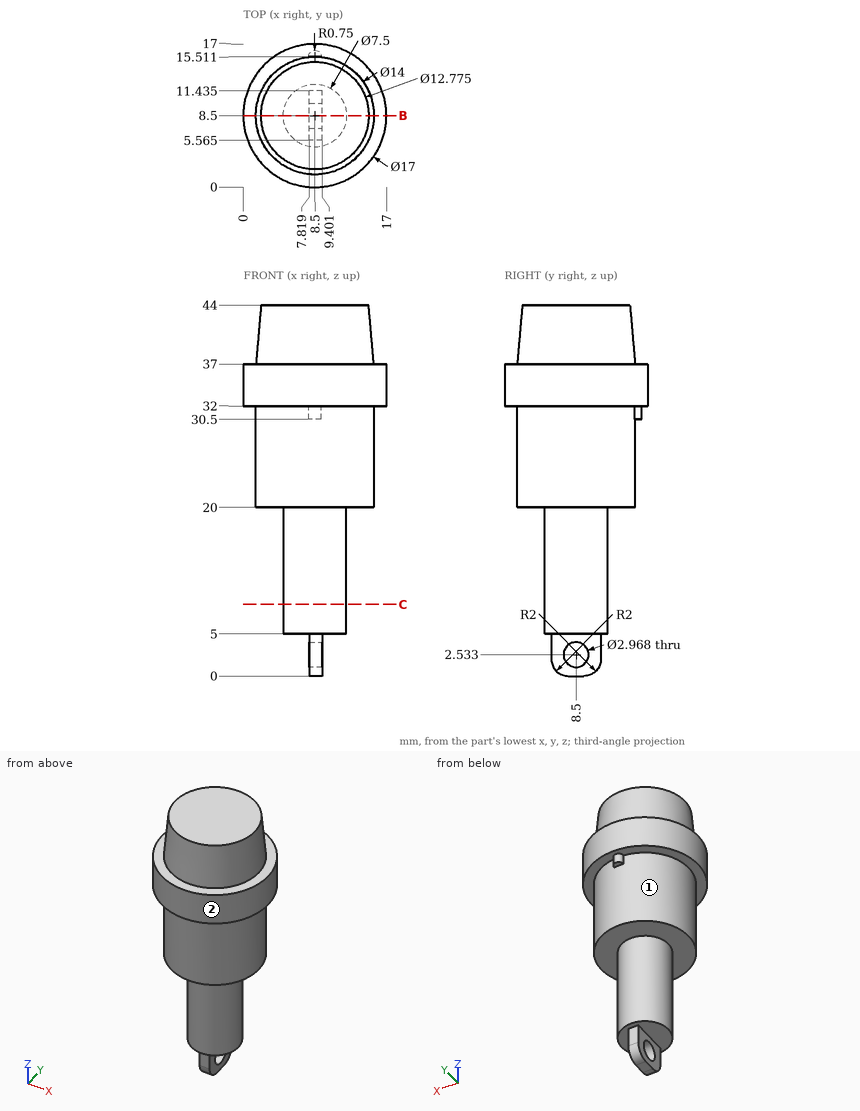
Print and shaded views of the part. All mm, measured from the part's lowest x, y and z. A direction names the side the tool comes from. Round coordinates to 2 decimals unless told otherwise and drop trailing zeros. Order: outer loops, then holes, each group sorted by start corner. A loop starts at its lowest first (then second) coordinate and runs counter-clockwise, first axis right, second up.
Q1. Drop flat-ended pins along their axis: pin 1 (10 mm diameter, centred on y = 12, z = 26.5, fed in from -X); pin 2 (3 mm diameter, centred on y = 5.5, z = 24.5, fed in from -X); pin 3 (4 mm diameter, centred on y = 8.5, z = 2, fed in from -X); pin 4 (1.5 mm diameter, centred on x = 13.5, z = 9.5, fed in from +Y). Give the stop position or say it passes through.
Q2. Slice it at B-B (y = 8.5). Write the cut outline in (x, z).
Q3. Which spindle directions (+Z, -Z, +X, -X, +Y, -Y) get a long thin tool onto all of the face, cutting with end or side? Do the marked faces 1 and 2. Say none if no direction does.
Q4. Slice it at C-C (z = 8.5). Write the cut outline in (x, y).
Q5. Wall check: L1, parallel to Z at x = 9.5, y = 15.5; L2, parallel to Z at x = 9, y = 3.5; L3, parallel to X at y = 8.25, z = 15.5. Give the ranges that are in metal, low to high.
Results below:
1. pin 1: stops at x = 1.5
1. pin 2: stops at x = 1.66
1. pin 3: stops at x = 7.82
1. pin 4: passes through
2. outline: (0, 32) - (1.5, 32) - (1.5, 20) - (4.75, 20) - (4.75, 5) - (7.82, 5) - (7.82, 4.02) - (9.4, 4.02) - (9.4, 5) - (12.25, 5) - (12.25, 20) - (15.5, 20) - (15.5, 32) - (17, 32) - (17, 37) - (15.5, 37) - (14.89, 44) - (2.11, 44) - (1.5, 37) - (0, 37) - close; (7.82, 0) - (9.4, 0) - (9.4, 1.05) - (7.82, 1.05) - close
3. face 1: -Z
3. face 2: +Z, -Z
4. outline: circle Ø7.5 at (8.5, 8.5)
5. L1: z = 32 to 37
5. L2: z = 20 to 44
5. L3: x = 4.76 to 12.24
